CAD build for the part. Positions are in the model's coordinates, mm. A direction names the side the tool comes from. Give positions to 0.01 mm unless a question says otherwise; leave off trailing zeros. Order: outer loops, then holes, each group sorted by start corner. A loop starts at its lowest first (then second) coordinate and runs counter-clockwise, first axis right, second up. Notation, with made-up numbers: (64.5, 47) -> (69.5, 47) arc R14 ccw to (69.5, 56) -> close; hole circle Ø9 at (63, -22.75). An arc over 180 degrees is marked (long way). Answer as CSV lines item,"result".
```python
from build123d import *

# Parameters (mm, degrees)
PAD_DEPTH            = 25
PAD001_DEPTH         = 18
SKETCH009_R          = 1.5
POCKET_DEPTH         = 22.037219
SKETCH010_W          = 4
SKETCH010_H          = 4
SKETCH010_W_2        = 10
POCKET001_DEPTH      = 6
POCKET002_DEPTH      = 0.001
POCKET002_DEPTH_BACK = -57.785827


with BuildPart() as part:
    # Sketch006 → Pad (new body, symmetric)
    with BuildSketch(Plane(origin=(32.784826, 3e-06, 0), x_dir=(0, 1, 0), z_dir=(1, 0, 0))):
        with BuildLine():
            Line((4, 0), (4, 15))
            add(Edge.make_bspline(
                [(4, 15), (4, 23.212807), (-14, 23.393326), (-22.61293, 10), (-22.61293, 7.866463)],
                knots=[0, 0, 0, 0, 0.5, 1, 1, 1, 1], degree=3))
            Line((-22.61293, 7.866463), (-19.793852, 6.840403))
            add(Edge.make_bspline(
                [(-3.8, 19.5), (-13.258017, 19), (-19.793852, 8.97394), (-19.793852, 6.840403)],
                knots=[0, 0, 0, 0, 1, 1, 1, 1], degree=3))
            ThreePointArc((-3.8, 19.5), (-1.55, 17.25), (-3.8, 15))
            Line((-3.8, 15), (-4, 15))
            Line((-4, 15), (-4, 1.091911))
            Line((-4, 1.091911), (-1, 0))
            Line((-1, 0), (4, 0))
        make_face()
    extrude(amount=PAD_DEPTH, both=True)

    # Sketch008 (on Face9 of Pad) → Pad001 (join)
    with BuildSketch(Plane(origin=(32.784826, 3e-06, 0), x_dir=(0, 1, 0), z_dir=(0, 0, -1))):
        Polygon((3.05, 6.5), (3.05, -6.5), (4.6, -4.95), (9.8, -4.65), (16, -1.4), (16, 1.4), (9.8, 4.65), (4.6, 4.95), align=None)
    extrude(amount=-PAD001_DEPTH)

    # Sketch009 (on Face5 of Pad001) → Pocket (cut, through all)
    with BuildSketch(Plane(origin=(32.784826, 3e-06, 0), x_dir=(0, 1, 0), z_dir=(0, 0, -1))):
        with Locations((0, -8)):
            Circle(SKETCH009_R)
        with Locations((0, 8)):
            Circle(SKETCH009_R)
        Polygon((-34, -26), (4, -26), (4, -12), (1.35, -24), (-0.5, -25), (-34, -22), align=None)
        Polygon((-34, 26), (4, 26), (4, 12), (1.35, 24), (-0.5, 25), (-34, 22), align=None)
    extrude(amount=-POCKET_DEPTH, mode=Mode.SUBTRACT)

    # Sketch010 (on Face12 of Pocket) → Pocket001 (cut)
    with BuildSketch(Plane(origin=(32.784826, 4.000003, 0), x_dir=(0, 0, 1), z_dir=(0, 1, 0))):
        with Locations((7.5, 8)):
            Rectangle(SKETCH010_W, SKETCH010_H)
        with Locations((7.5, -8)):
            Rectangle(SKETCH010_W, SKETCH010_H)
        with Locations((20, 8)):
            Rectangle(SKETCH010_W_2, SKETCH010_H)
        with Locations((20, -8)):
            Rectangle(SKETCH010_W_2, SKETCH010_H)
    extrude(amount=-POCKET001_DEPTH, mode=Mode.SUBTRACT)

    # Sketch → Pocket002 (cut, two sides)
    with BuildSketch(Plane.YZ) as pocket002_sk:
        Polygon((11, 19), (16.940921, 19), (16.940921, 16.837682), align=None)
        Polygon((12.734107, -0.552658), (17, -0.552658), (17, 1), align=None)
    extrude(amount=-POCKET002_DEPTH, mode=Mode.SUBTRACT)
    extrude(pocket002_sk.sketch, amount=-POCKET002_DEPTH_BACK, mode=Mode.SUBTRACT)


solid = part.part
```
1) Band-saw the part on B-B, the plane y = 9. Write the cut outline in (x, z), then the cut area to 3 significant figures.
Data:
outline,"(28.09, 0) -> (37.48, 0) -> (37.48, 18) -> (28.09, 18) -> close"
area,"169 mm2"
2) Which spindle directions (+Z, -Z, +X, -X, +Y, -Y) get a long thin tool onto all of the face, cutting with end or side? Do faces 4 (the flat face through (38.785, 1, 7)), 5 (the flat face through (25, -2, 20)), 6 (the flat face through (57.3, 0.4, 10.7)). Say none if no direction does.
Data:
face 4,"+Y"
face 5,"+Z, +Y"
face 6,"+Z, -Z, +X, +Y"
3) Pin check, flat tips, straight feed: P1, Ø1.7, axis at x = 25, z = 20.5, coming from the +Y side; P2, Ø8, axis at x = 34, y = 8, coming from the +Z side; P3, Ø12, axis at y = -5.5, z = 5.5, coming from the -X side. Stop position of each tip, or through.
Data:
P1,"stops at y = -2"
P2,"stops at z = 18"
P3,"stops at x = 7.78"
4) Band-saw the part on A-A, the plane z = 3. Write the cut outline in (x, y).
Data:
outline,"(7.78, -0.5) -> (8.1, -4) -> (57.47, -4) -> (57.78, -0.5) -> (56.78, 1.35) -> (44.78, 4) -> (38.33, 4) -> (37.73, 4.6) -> (37.43, 9.8) -> (34.18, 16) -> (31.38, 16) -> (28.13, 9.8) -> (27.83, 4.6) -> (27.23, 4) -> (20.78, 4) -> (8.78, 1.35) -> close; hole circle Ø3 at (24.78, 0); hole circle Ø3 at (40.78, 0)"
5) Wall check: line 1 along Y through (x, z) = (25, 13.25); line 2 along X through (y, z) = (1, 19); line 3 along Y through (x, z) = (13.5, 12.5). Give the ranges that are in metal, low to high. Write a range as [from, to].
Data:
line 1,"y = [-19.82, -15.86], [-4, -1.48], [1.48, 4]"
line 2,"x = [8.6, 22.78], [26.78, 38.78], [42.78, 56.97]"
line 3,"y = [-20.39, -16.53], [-4, 2.39]"
6) Pull direction X, two halves, no side cores. Call faces 1 (the flat face through (41, -2, 7)), 2 (the flat face through (8.037, -3.315, 13.423)), 3 (the flat face through (22.6, 4, 7.4)): pulls with the +X half, pulls with the -X half, needs draft (parallel to the pull), parting line crosses it, or undercut.
Data:
face 1,"undercut"
face 2,"pulls with the -X half"
face 3,"needs draft"
